Build history of the part. All positions in model axes, mm. A direction names the side the tool comes from. Give positions to 0.01 mm unless a question says otherwise; leave off trailing zeros. Order: outer loops, then holes, each group sorted by start corner. A loop starts at its lowest first (then second) coordinate and runs counter-clockwise, first axis right, second up. Notation, with made-up numbers: M 80.25,-35.75 L 93.25,-35.75 A11 cw 93.25,-25.75 Z; hole C 74,-2.5 d10. An arc over 180 degrees is marked long. One line per item, written item: value.
from build123d import *

# Parameters (mm, degrees)
SKETCH1_R           = 30.5
BOSS_EXTRUDE1_DEPTH = 26.1
SKETCH2_R           = 10.25
BOSS_EXTRUDE2_DEPTH = 3
SKETCH3_R           = 17.25
BOSS_EXTRUDE3_DEPTH = 7.2
CUT_EXTRUDE1_START  = -10.2
CUT_EXTRUDE1_DEPTH  = 10.2
SKETCH4_4_R         = 1.5
CUT_EXTRUDE2_DEPTH  = 7.2
SKETCH7_R           = 4
BOSS_EXTRUDE4_DEPTH = 55.5
FILLET1_R           = 1.25
SKETCH8_R           = 1.55
BOSS_EXTRUDE5_DEPTH = 8.175


# Read off the part's stored shape, not the designer's step: M8x1.25 Machine Threads Stud1
with BuildPart() as part:
    # Sketch1 → Boss-Extrude1 (new body)
    with BuildSketch(Plane(origin=(0, 0, 0), x_dir=(1, 0, 0), z_dir=(0, 1, 0))):
        with Locations(Location((0, 0, 0), (0, 0, 270))):
            Circle(SKETCH1_R)
    extrude(amount=BOSS_EXTRUDE1_DEPTH)

    # Sketch2 → Boss-Extrude2 (add)
    with BuildSketch(Plane(origin=(0, 26.1, 0), x_dir=(1, 0, 0), z_dir=(0, 1, 0))):
        with Locations(Location((0, 0, 0), (0, 0, 270))):
            Circle(SKETCH2_R)
    extrude(amount=BOSS_EXTRUDE2_DEPTH)

    # Sketch3 → Boss-Extrude3 (add)
    with BuildSketch(Plane(origin=(0, 29.1, 0), x_dir=(1, 0, 0), z_dir=(0, 1, 0))):
        with Locations(Location((0, 0, 0), (0, 0, 270))):
            Circle(SKETCH3_R)
    extrude(amount=BOSS_EXTRUDE3_DEPTH)

    # Sketch4 → Cut-Extrude1 (cut)
    with BuildSketch(Plane(origin=(0, 36.3, 0), x_dir=(1, 0, 0), z_dir=(0, 1, 0)).offset(CUT_EXTRUDE1_START)):
        with BuildLine():
            ThreePointArc((-13.966070745, -5.472555887), (-12.990381057, 7.5), (-2.243662951, 14.83125))
            ThreePointArc((-2.243662951, 14.83125), (-1.649573809, 16.530165432), (0, 17.25))
            ThreePointArc((0, 17.25), (-14.938938189, 8.625000045), (-14.938938267, -8.62499991))
            ThreePointArc((-14.938938267, -8.62499991), (-15.140330082, -6.836509843), (-13.966070745, -5.472555887))
        make_face()
        with BuildLine():
            ThreePointArc((2.243662951, 14.83125), (12.990381057, 7.5), (13.966070745, -5.472555887))
            ThreePointArc((13.966070745, -5.472555887), (15.140330099, -6.836509898), (14.938938209, -8.62500001))
            ThreePointArc((14.938938209, -8.62500001), (14.938938218, 8.624999995), (0, 17.25))
            ThreePointArc((0, 17.25), (1.649573809, 16.530165432), (2.243662951, 14.83125))
        make_face()
        with BuildLine():
            ThreePointArc((11.722407794, -9.358694113), (0, -15), (-11.722407794, -9.358694113))
            ThreePointArc((-11.722407794, -9.358694113), (-13.49075634, -9.693655528), (-14.938938267, -8.62499991))
            ThreePointArc((-14.938938267, -8.62499991), (-5.8e-08, -17.25), (14.938938209, -8.62500001))
            ThreePointArc((14.938938209, -8.62500001), (13.490756283, -9.693655541), (11.722407794, -9.358694113))
        make_face()
    extrude(amount=CUT_EXTRUDE1_DEPTH, mode=Mode.SUBTRACT)

    # Sketch4<4> → Cut-Extrude2 (cut)
    with BuildSketch(Plane(origin=(0, 36.3, 0), x_dir=(1, 0, 0), z_dir=(0, 1, 0))):
        with Locations(Location((0, 15, 0), (0, 0, 270))):
            Circle(SKETCH4_4_R)
        with Locations(Location((12.990381057, -7.5, 0), (0, 0, 270))):
            Circle(SKETCH4_4_R)
        with Locations(Location((-12.990381057, -7.5, 0), (0, 0, 270))):
            Circle(SKETCH4_4_R)
    extrude(amount=-CUT_EXTRUDE2_DEPTH, mode=Mode.SUBTRACT)

    # Sketch7 → Boss-Extrude4 (add)
    with BuildSketch(Plane(origin=(0, 36.3, 0), x_dir=(1, 0, 0), z_dir=(0, 1, 0))):
        with Locations(Location((0, 0, 0), (0, 0, 270))):
            Circle(SKETCH7_R)
    extrude(amount=BOSS_EXTRUDE4_DEPTH)

    # Fillet1
    fillet1_edges = [part.edges().sort_by_distance(p)[0] for p in [
        (0, 0, -30.5),
        (-13.966070745, 32.7, 5.472555887),
        (-2.243662951, 32.7, -14.83125),
        (13.966070745, 32.7, 5.472555887),
        (2.243662951, 32.7, -14.83125),
        (-11.722407794, 32.7, 9.358694113),
        (11.722407794, 32.7, 9.358694113),
    ]]
    fillet(fillet1_edges, radius=FILLET1_R)

    # Sketch8 → Boss-Extrude5 (add, symmetric)
    with BuildSketch(Plane.XY):
        with Locations(Location((0, 60.5, 0), (0, 0, 180))):
            Circle(SKETCH8_R)
    extrude(amount=BOSS_EXTRUDE5_DEPTH, both=True)

    # M8x1.25 Machine Threads Stud1 outline → M8x1.25 Machine Threads Stud1 (revolve, cut)
    with BuildSketch(Plane.XY):
        Polygon((4, 91.8), (3.3095, 91.8), (4, 91.1095), align=None)
    revolve(axis=Axis((0, 0, 0), (0, 1, 0)), mode=Mode.SUBTRACT)


solid = part.part
1) Tool access for faces 5 (the face through (0.07, 32.75, -16.5)), 6 (the face through (-13.077, 32.65, -7.347)), 7 (the face through (1.55, 60.43, -5.9)): list every direction of +Z, -Z, +X, -X, +Y, -Y with a clear straight run to the whole face (end or side of a thin tool).
Check values:
face 5: +Y
face 6: -X, +Y
face 7: -Z
2) Pin check, flat tips, straight feed: pin 1 (1.8 mm diameter, centred on x = 0, z = -15, fed in from +Y); pin 2 (6 mm diameter, centred on x = 0, y = 29.5, fed in from +Z); pin 3 (3.5 mm diameter, centred on x = 0.5, y = 61, fed in from -Z) (3 decimals). Stop position of each tip, or through.
Check values:
pin 1: y = 26.1
pin 2: z = 15
pin 3: z = -8.175
3) Saw through at B-B, the plane z = 0. Write the cut outline in (x, y), then the cut area to 3 significant figures.
Check values:
outline: M -30.5,1.25 A1.25 ccw -29.25,0 L 29.25,0 A1.25 ccw 30.5,1.25 L 30.5,26.1 L 10.25,26.1 L 10.25,29.1 L 15,29.1 L 15,36.3 L 4,36.3 L 4,91.11 L 3.31,91.8 L -3.31,91.8 L -4,91.11 L -4,36.3 L -15,36.3 L -15,29.1 L -10.25,29.1 L -10.25,26.1 L -30.5,26.1 Z
area: 2,310 mm^2
4) Mould opens along Z. For faces 1 (the face through (0, 33, 15)), 2 (the face through (-13, 26.1, 0)), 3 (the face through (-13, 33, 6)), 4 (the face through (-29.775, 13.501, -6.612)) say: released by +Z, released by -Z, zero draft, split by the parting line, or undercut.
Check values:
face 1: released by +Z
face 2: zero draft
face 3: undercut
face 4: split by the parting line
5) Saw through at A-A, the plane y = 60.5. Write the cut outline in (x, z) (3 decimals).
Check values:
outline: M -1.55,-8.175 L 1.55,-8.175 L 1.55,-3.687 A4 ccw 1.55,3.687 L 1.55,8.175 L -1.55,8.175 L -1.55,3.687 A4 ccw -1.55,-3.687 Z
6) Drill centre lines: probe 1 along X at (y, z) = (33.5, 7.5); probe 2 along X at (y, z) = (31, 7); probe 3 along Y at (x, z) = (-16, -18.5). Where is each one in solid material? Low to high. Write a range as from..to.
Check values:
probe 1: -15.24..-14.49, -11.49..11.49, 14.49..15.24
probe 2: -15.18..-14.4, -11.58..11.58, 14.4..15.18
probe 3: 0..26.1
